Verification items for the finished model (mm, model axes). Face numbers are marked on the shaded views. A direction names the side the tool comes from. Round coordinates to 2 decimals unless told otherwise and drop trailing zeros. Write each loop counter-clockwise with the first axis right and the second up, starting at its lowest first coordinate (ties: lowest second). Pieces come first, ordered by that corner, then holes. Notation, with made-up numbers: (-12, 27.5) - (38, 27.5) arc R28 cw to (38, 49.5) - close; hole circle Ø10 at (-39, 35.25). An arc over 180 degrees is marked (long way). Answer as a JSON object with one key per item and string values.
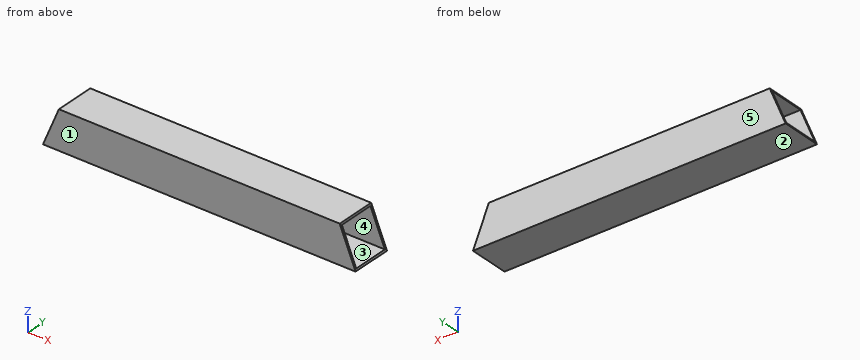
```python
from build123d import *

# Parameters (mm, degrees)
BOSS_EXTRUDE1_DEPTH = 1.2
BOSS_EXTRUDE2_START = 25.4
BOSS_EXTRUDE2_DEPTH = 1.2
BOSS_EXTRUDE3_DEPTH = 24.2


with BuildPart() as part:
    # Sketch1 → Boss-Extrude1 (new body)
    with BuildSketch(Plane(origin=(0, 0, 0), x_dir=(1, 0, 0), z_dir=(0, 1, 0))):
        Polygon((-103.553390593, 250), (-93.032366109, 224.6), (93.032366109, 224.6), (103.553390593, 250), align=None)
    extrude(amount=BOSS_EXTRUDE1_DEPTH)



with BuildPart() as body_2:
    # Sketch2 → Boss-Extrude2 (new body)
    with BuildSketch(Plane(origin=(0, 1.2, 0), x_dir=(1, 0, 0), z_dir=(0, 1, 0)).offset(BOSS_EXTRUDE2_START)):
        Polygon((93.032366109, 224.6), (103.553390593, 250), (-103.553390593, 250), (-93.032366109, 224.6), align=None)
    extrude(amount=-BOSS_EXTRUDE2_DEPTH)


with BuildPart() as part_1:
    add(part.part)

    add(body_2.part)  # Boss-Extrude3 merges body 2
    # Sketch3 → Boss-Extrude3 (add)
    with BuildSketch(Plane(origin=(0, 1.2, 0), x_dir=(1, 0, 0), z_dir=(0, 1, 0))):
        Polygon((93.032366109, 224.6), (93.529422384, 225.8), (-93.529422384, 225.8), (-93.032366109, 224.6), align=None)
        Polygon((-103.553390593, 250), (-103.056334318, 248.8), (103.056334318, 248.8), (103.553390593, 250), align=None)
    extrude(amount=BOSS_EXTRUDE3_DEPTH)


solid = part_1.part
```
Q1. Section check C-C, the plane x = 22. Record the cut outline in (y, z).
Geometry check:
{"outline": "(0, -250) - (26.6, -250) - (26.6, -224.6) - (0, -224.6) - close; hole (1.2, -248.8) - (25.4, -248.8) - (25.4, -225.8) - (1.2, -225.8) - close"}
Q2. Section check B-B, the plane z = -238.25. Record the cut outline in (x, y).
Geometry check:
{"outline": "(-98.69, 0) - (98.69, 0) - (98.69, 1.2) - (-98.69, 1.2) - close; (-98.69, 25.4) - (98.69, 25.4) - (98.69, 26.6) - (-98.69, 26.6) - close"}
Q3. Section check A-A, the plane y = 17.5. Record the cut outline in (x, z).
Geometry check:
{"outline": "(-103.55, -250) - (103.55, -250) - (103.06, -248.8) - (-103.06, -248.8) - close; (-93.53, -225.8) - (93.53, -225.8) - (93.03, -224.6) - (-93.03, -224.6) - close"}
Q4. Release check for a two-part mould opening along Y. For the marked faces 1, 2 and 3 record: released by +Y, released by -Y, zero draft, split by the parting line, or undercut.
Geometry check:
{"face 1": "released by -Y", "face 2": "zero draft", "face 3": "undercut"}
Q5. Set-up check for the marked faces 4 and 5: record each of +Z, -Z, +X, -X, +Y, -Y from which the full face is reachable in a straight line by a thin tool's end or side.
Geometry check:
{"face 4": "+X, -X", "face 5": "+Z, -Z, +X, -X, +Y"}
Q6. Material ranges on line 1 along Z through (x, y) = (26, 24.75); line 2 along Y through (x, z) = (31.5, -241), recorded low to high. Write a range as [from, to].
Geometry check:
{"line 1": "z = [-250, -248.8], [-225.8, -224.6]", "line 2": "y = [0, 1.2], [25.4, 26.6]"}
Q7. Gauge pin test, flat end, axial feed: P1, Ø12, axis at y = 10.5, z = -229.5, coming from the +X side. Record the tip position at first contact, or that the pin passes through.
Geometry check:
{"P1": "stops at x = 93.53"}
